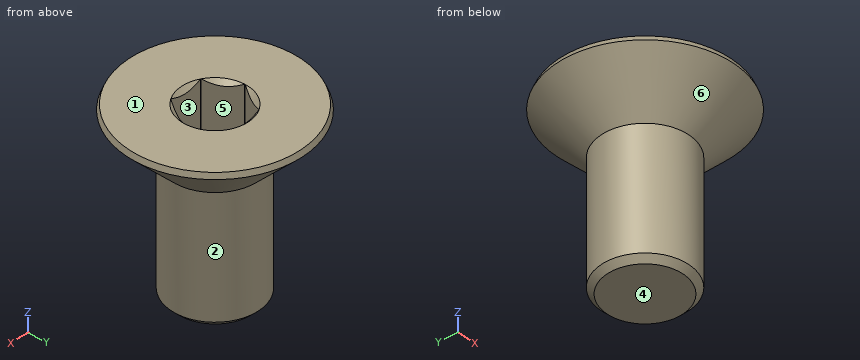
```python
from build123d import *

# Parameters (mm, degrees)
SKETCH001_R     = 2.15
POCKET_DEPTH    = 3.119566
CHAMFER_SIZE    = 0.25
CHAMFER001_SIZE = 0.2


with BuildPart() as pocket:
    # Sketch003 → Revolution001 (revolve)
    with BuildSketch(Plane.XZ):
        Polygon((0, -2.118566), (1.15, -1.7), (1.15, 1), (0, 1), align=None)
    revolve(axis=Axis((0, 0, 0), (0, 0, 1)))

    # Sketch001 → Pocket (cut, through all)
    with BuildSketch(Plane(origin=(0, 0, 1), x_dir=(-1, 0, 0), z_dir=(0, 0, 1))):
        Circle(SKETCH001_R)
        Polygon((-0.57735, 1), (0.57735, 1), (1.154701, 0), (0.57735, -1), (-0.57735, -1), (-1.154701, 0), align=None, mode=Mode.SUBTRACT)
    extrude(amount=-POCKET_DEPTH, mode=Mode.SUBTRACT)


with BuildPart() as chamfer001:
    # Sketch → Revolution (revolve)
    with BuildSketch(Plane.XZ):
        Polygon((1.15, 0), (3.199999, 0), (1.5, -1.7), (1.5, -6), (0, -6), (0, -1.150001), align=None)
    revolve(axis=Axis((0, 0, 0), (0, 0, 1)))

    # Cut: cut Pocket
    add(pocket.part, mode=Mode.SUBTRACT)

    # Chamfer
    chamfer_edges = [chamfer001.edges().sort_by_distance(p)[0] for p in [
        (-3.199999, 0, 0),
    ]]
    chamfer(chamfer_edges, length=CHAMFER_SIZE)

    # Chamfer001
    chamfer001_edges = [chamfer001.edges().sort_by_distance(p)[0] for p in [
        (-1.5, 0, -6),
    ]]
    chamfer(chamfer001_edges, length=CHAMFER001_SIZE)


solid = chamfer001.part
```
Input: part model. Units: mm. Frame: model coordinates. Face numbers are marked on the shaded views. A direction names the side the tool comes from. Give positions to 0.01 mm unless a question says otherwise; leave off trailing zeros. Loops run counter-clockwise (first coordinate to the right, second up) from the corner with the lowest first, then second, coordinate; pieces in that order, holes last. Notation, with made-up numbers: (7, 32.25) -> (29, 32.25) arc R20 ccw to (29, 58.25) -> close; hole circle Ø11 at (-36, 11.25). An arc over 180 degrees is marked (long way). Use a Markdown table: item, result.
Q1. First-contact query: P1, Ø2, axis at x = -0.5, y = 0.5, coming from the +Z side; P2, Ø2, axis at y = -0.5, z = -5, coming from the -X side; P3, Ø0.9, axis at x = 0, z = -1, coming from the -Y side; P4, Ø1, axis at x = -2, z = -1, coming from the +Y side. Flat tips, straight axial feed; report the tip coordinate or a pass-through.
Entries:
| item | result |
|---|---|
| P1 | stops at z = 0 |
| P2 | stops at x = -1.5 |
| P3 | stops at y = -2.65 |
| P4 | stops at y = 1.97 |
Q2. Access query for the marked faces 1 and 2. Directions: +Z, -Z, +X, -X, +Y, -Y. A direction counts if a zero-diameter tool reaches every point of the face in a straight line with its end or side. Return the directions, or none.
Entries:
| item | result |
|---|---|
| face 1 | +Z, +X, -X, +Y, -Y |
| face 2 | -Z |
Q3. Section query B-B, the plane z = -3.2. Return the cut outline in (x, y), plus the area to 3 significant figures.
Entries:
| item | result |
|---|---|
| outline | circle Ø3 at (0, 0) |
| area | 7.07 mm² |
Q4. Ray query, probe 1 along Y at (x, z) = (-0.75, -0.4); probe 2 along Y at (x, z) = (-0.5, -0.3); probe 3 along Z at (x, y) = (-1, -2). Return the intervals inside material, ascending. Write a range as from..to.
Entries:
| item | result |
|---|---|
| probe 1 | y = -2.7..-0.7, 0.7..2.7 |
| probe 2 | y = -2.86..-1, 1..2.86 |
| probe 3 | z = -0.96..0 |
Q5. Pull-direction query (Y, two-part tool) for the marked faces 3, 4, 5 and 6; classes: pulls with the +Y half, pulls with the -Y half, needs draft (parallel to the pull), parting line crosses it, or undercut.
Entries:
| item | result |
|---|---|
| face 3 | undercut |
| face 4 | needs draft |
| face 5 | undercut |
| face 6 | parting line crosses it |
